CAD build for the part. Positions are in the model's coordinates, mm. A direction names the side the tool comes from. Give positions to 0.01 mm unless a question says otherwise; leave off trailing zeros. Loops run counter-clockwise (first coordinate to the right, second up) from the corner with the lowest first, then second, coordinate; pieces in that order, holes last.
Item 1: Saw through at A-A on x = 36.5. Give the cut face in (y, z) (3 decimals), plus the area to 3 significant figures.
Item 2: Probe probe 1 along X at (y, z) = (7.25, -1); probe 2 along X at (y, z) = (6.25, -5); probe 3 along Y at (x, z) = (36.5, -2.25) (3 decimals). List the from-to ranges inside material, lowest first.
Item 3: Mould opens along X. For faces 1 (the flat face through (91.5, 5.3, -3.62)), 2 (the cylindrical face through (105.586, 0.724, -4.37)), 3 (the flat face through (61, 14, 0)) say: released by +X, released by -X, zero draft, split by the parting line, or undercut.
Item 4: Which spindle directions (+Z, -Z, +X, -X, +Y, -Y) get a long thin tool onto all of the face, cutting with end or side? Do faces 4 (the flat face through (29, 5, -3.62)), 5 (the flat face through (61, 28.575, -4)). Say none if no direction does.
Item 5: Saw through at B-B on y = 21.25. Give the cut face in (x, z), plus the area to 3 significant figures.
Item 6: Drop flat-ended pins along their axis: P1, Ø5, axis at x = 93.225, y = 7, coming from the +Z side; P2, Ø3.5, axis at x = 31.075, y = 7, coming from the -Z side; P3, Ø2.5, axis at x = 93, y = 5.5, coming from the -Z side. Give the stop position or say it passes through.
Item 7: Saw through at D-D on x = 93. Give the cut face in (y, z) (3 decimals), plus the area to 3 significant figures.
Item 8: Saw through at C-C on z = -2. Give the cut face in (x, y) (3 decimals), plus the area to 3 significant figures.
from build123d import *

# Parameters (mm, degrees)
SKETCH1_W                      = 88.9
SKETCH1_H                      = 15.875
BOSS_EXTRUDE1_DEPTH            = 7.62
CBORE_FOR_M4_SHCS1_D           = 4.5
CBORE_FOR_M4_SHCS1_CBORE_D     = 8
CBORE_FOR_M4_SHCS1_CBORE_DEPTH = 4
SKETCH4_W                      = 88.9
SKETCH4_H                      = 15.875
SKETCH4_R                      = 4
BOSS_EXTRUDE2_DEPTH            = 1
SKETCH5_W                      = 88.9
SKETCH5_H                      = 12.7
SKETCH5_R                      = 2
BOSS_EXTRUDE3_DEPTH            = 8.62
M4_CLEARANCE_HOLE1_D           = 4.5
FILLET1_R                      = 2.54


with BuildPart() as part:
    # Sketch1 → Boss-Extrude1 (new body)
    with BuildSketch(Plane.XY):
        with Locations((61.9, 7.9375)):
            Rectangle(SKETCH1_W, SKETCH1_H)
    extrude(amount=-BOSS_EXTRUDE1_DEPTH)

    # CBORE for M4 SHCS1 (through all)
    with Locations(Plane(origin=(0, 0, -7.62), x_dir=(-1, 0, 0), z_dir=(0, 0, -1))):
        with Locations((-93.225, 7), (-31.075, 7)):
            CounterBoreHole(CBORE_FOR_M4_SHCS1_D / 2, CBORE_FOR_M4_SHCS1_CBORE_D / 2, CBORE_FOR_M4_SHCS1_CBORE_DEPTH)

    # Sketch4 → Boss-Extrude2 (add)
    with BuildSketch(Plane(origin=(0, 0, -7.62), x_dir=(-1, 0, 0), z_dir=(0, 0, -1))):
        with Locations((-61.9, 7.9375)):
            Rectangle(SKETCH4_W, SKETCH4_H)
        with Locations((-93.225, 7)):
            Circle(SKETCH4_R, mode=Mode.SUBTRACT)
        with Locations((-31.075, 7)):
            Circle(SKETCH4_R, mode=Mode.SUBTRACT)
    extrude(amount=BOSS_EXTRUDE2_DEPTH)

    # Sketch5 → Boss-Extrude3 (add)
    with BuildSketch(Plane.XY):
        with Locations((61.9, 22.225)):
            Rectangle(SKETCH5_W, SKETCH5_H)
        with Locations((36.5, 22.225)):
            Circle(SKETCH5_R, mode=Mode.SUBTRACT)
        with Locations((87.3, 22.225)):
            Circle(SKETCH5_R, mode=Mode.SUBTRACT)
        with Locations((36.5, 22.225)):
            Circle(SKETCH5_R)
        with Locations((87.3, 22.225)):
            Circle(SKETCH5_R)
    extrude(amount=-BOSS_EXTRUDE3_DEPTH)

    # M4 Clearance Hole1 (through all)
    with Locations(Plane.XY):
        with Locations((36.5, 22.225), (87.3, 22.225)):
            Hole(M4_CLEARANCE_HOLE1_D / 2)

    # Fillet1
    fillet1_edges = [part.edges().sort_by_distance(p)[0] for p in [
        (17.45, 28.575, -4.31),
        (106.35, 28.575, -4.31),
        (106.35, 0, -4.31),
        (17.45, 0, -4.31),
    ]]
    fillet(fillet1_edges, radius=FILLET1_R)


solid = part.part
Results below:
1. outline: (0, -8.62) - (19.975, -8.62) - (19.975, 0) - (0, 0) - close; (24.475, -8.62) - (28.575, -8.62) - (28.575, 0) - (24.475, 0) - close
1. area: 208 mm2
2. probe 1: x = 17.45 to 28.84, 33.31 to 90.99, 95.46 to 106.35
2. probe 2: x = 17.45 to 27.15, 35 to 89.3, 97.15 to 106.35
2. probe 3: y = 0 to 19.975, 24.475 to 28.575
3. face 1: undercut
3. face 2: released by +X
3. face 3: zero draft
4. face 4: -Z
4. face 5: +Z, -Z, +X, -X, +Y
5. outline: (17.45, -8.62) - (34.47, -8.62) - (34.47, 0) - (17.45, 0) - close; (38.53, -8.62) - (85.27, -8.62) - (85.27, 0) - (38.53, 0) - close; (89.33, -8.62) - (106.35, -8.62) - (106.35, 0) - (89.33, 0) - close
5. area: 696 mm2
6. P1: stops at z = 0
6. P2: passes through
6. P3: stops at z = -3.62
7. outline: (0, -8.62) - (3.006, -8.62) - (3.006, -3.62) - (4.761, -3.62) - (4.761, 0) - (0, 0) - close; (9.239, -3.62) - (10.994, -3.62) - (10.994, -8.62) - (28.575, -8.62) - (28.575, 0) - (9.239, 0) - close
7. area: 190 mm2
8. outline: (17.45, 2.54) arc R2.54 ccw to (19.99, 0) - (103.81, 0) arc R2.54 ccw to (106.35, 2.54) - (106.35, 26.035) arc R2.54 ccw to (103.81, 28.575) - (19.99, 28.575) arc R2.54 ccw to (17.45, 26.035) - close; hole circle Ø4.5 at (31.075, 7); hole circle Ø4.5 at (36.5, 22.225); hole circle Ø4.5 at (87.3, 22.225); hole circle Ø4.5 at (93.225, 7)
8. area: 2,470 mm2
